Here's the drawing with two shaded views (mm, measured from the low corner). I have some questions. A direction names the side the tool comes from. Round coordinates to 2 decimals unless told otherwise and drop trailing zeros. Order: outer loops, then holes, each group sorted by start corner. A loop starts at its lowest first (then second) coordinate and runs counter-clockwise, first axis right, second up. Notation, with made-up numbers: (4.5, 74) -> (24.5, 74) arc R27 ccw to (24.5, 112) -> close; hole circle Ø4 at (46, 81.5). An arc over 180 degrees is marked (long way). Use a Markdown table: item, result. Add a question column.
Q1. If we section it at A-A on y = 13: List the corners of the cut face in (x, z) for me, plus the area to 3 significant figures.
Q2. I need wall thicknesses on line 1 along X through (y, z) = (48, 38); line 2 along X through (y, z) = (37.5, 6.5); line 3 along Z through (x, y) = (5.5, 48.5). Which ranges of each line are inside material? Lowest first, please. Write a range as [from, to].
Q3. If we section it at C-C on z = 29.5: List the corners of the cut face in (x, y) for me, plus the area to 3 significant figures.
Q4. For the marked faces 1 and 2, which set-ups out of +Z, -Z, +X, -X, +Y, -Y let a thin tool reach every point of the face, with its end or its side?
Q5. If we section it at B-B on x = 15.5: List the corners of the cut face in (y, z) for me, plus the area to 3 significant figures.
Q6. I'm going to push flat-ended pins straight in: pin 1 Ø8.5 at (y, z) = (22.5, 36) entering from -X; pin 2 Ø4 at (y, z) = (43, 24) entering from -X; pin 3 Ø10 at (y, z) = (10.5, 22.5) entering from -X. Where does each tip first touch, or does it pass through?
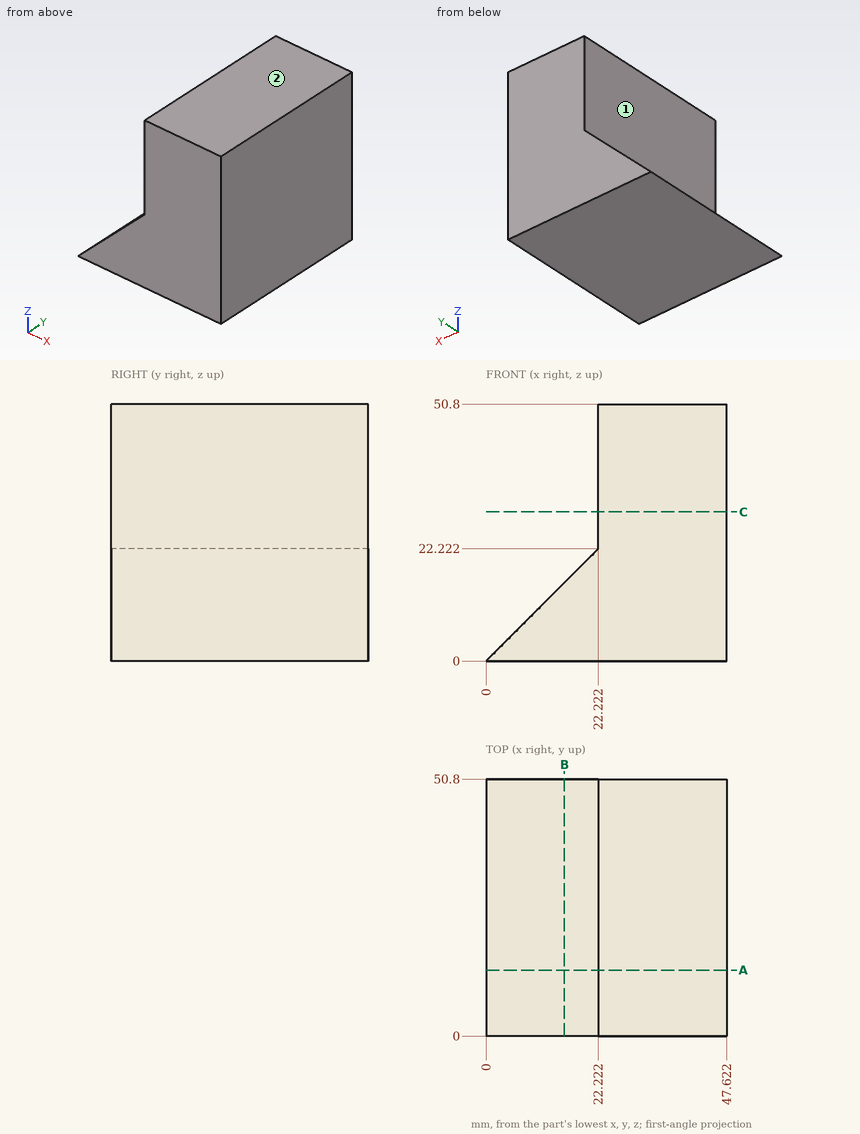
Answer below:
| question | item | result |
|---|---|---|
| 1 | outline | (0, 0) -> (47.62, 0) -> (47.62, 50.8) -> (22.22, 50.8) -> (22.22, 22.22) -> close |
| 1 | area | 1,540 mm² |
| 2 | line 1 | [22.22, 47.62] |
| 2 | line 2 | [6.5, 47.62] |
| 2 | line 3 | [0, 5.5] |
| 3 | outline | (22.22, 0) -> (47.62, 0) -> (47.62, 50.8) -> (22.22, 50.8) -> close |
| 3 | area | 1,290 mm² |
| 4 | face 1 | +Z, -X, +Y, -Y |
| 4 | face 2 | +Z, +X, -X, +Y, -Y |
| 5 | outline | (0, 0) -> (50.8, 0) -> (50.8, 15.5) -> (0, 15.5) -> close |
| 5 | area | 787 mm² |
| 6 | pin 1 | x = 22.22 |
| 6 | pin 2 | x = 22 |
| 6 | pin 3 | x = 17.5 |
